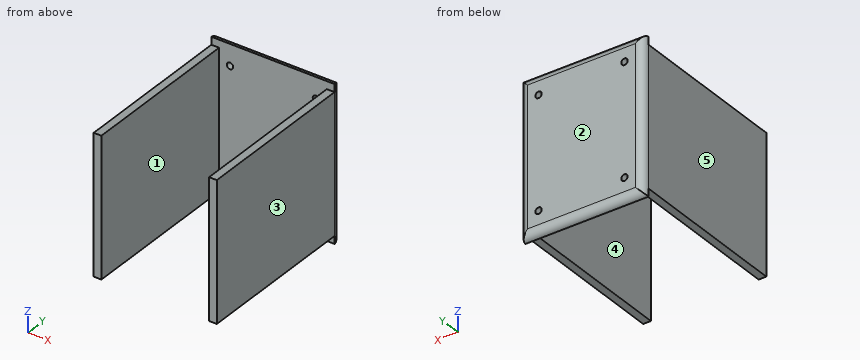
Autodesk Inventor part; units mm, degrees
ref_plane "YZ Plane" through (0, 0, 0) normal (1, 0, 0) x (0, 1, 0)
ref_plane "XZ Plane" through (0, 0, 0) normal (0, 1, 0) x (-1, 0, 0)
ref_plane "XY Plane" through (0, 0, 0) normal (0, 0, 1) x (1, 0, 0)
ref_plane "Plano de trabajo1" through (0, 3, 0) normal (0, 1, 0) x (1, 0, 0)
ref_plane "Plano de trabajo2" through (4.2498, 73, -5.25) normal (0, 1, 0) x (1, 0, 0)
sketch "Boceto3" plane through (4.2498, 73, -5.25) normal (0, 1, 0) x (1, 0, 0)
  line L0 (37.7502, 51.75) -> (40.7502, 51.75)
  line L1 (-7.2498, -8.25) -> (40.7502, -8.25)
  line L2 (40.7502, -8.25) -> (40.7502, 51.75)
  line L3 (40.7502, 51.75) -> (-7.2498, 51.75)
  line L4 (-7.2498, 51.75) -> (-7.2498, -8.25)
  circle A0 centre (33.5, 43.5) radius 1.25
  circle A1 centre (33.5, 0) radius 1.25
  circle A2 centre (0, 43.5) radius 1.25
  circle A3 centre (0, 0) radius 1.25
  point P0 (-4.2498, -5.25)
  point P1 (37.7502, -5.25)
  point P2 (37.7502, 48.75)
  dimension "d39" = 2.5
  dimension "d40" = 2.5
  dimension "d41" = 2.5
  dimension "d42" = 2.5
ref_plane "Plano de trabajo3" through (4.2498, 73, -5.25) normal (0, -1, 0) x (1, 0, 0)
sketch "Boceto5" plane through (4.2498, 73, -5.25) normal (0, -1, 0) x (1, 0, 0)
  line L0 (-4.2498, 5.25) -> (-4.2498, -48.75)
  line L1 (-4.2498, 5.25) -> (-4.2498, -48.75)
  line L2 (37.7502, -48.75) -> (37.7502, 5.25)
  line L3 (37.7502, 5.25) -> (37.7502, 8.25)
  line L4 (37.7502, -48.75) -> (37.7502, -51.75)
  line L5 (-4.2498, 5.25) -> (-7.2498, 5.25)
  line L6 (-4.2498, -48.75) -> (-7.2498, -48.75)
  line L7 (37.7502, -48.75) -> (40.7502, -48.75)
  line L8 (37.7502, 5.25) -> (40.7502, 5.25)
  line L9 (40.7502, 5.25) -> (40.7502, -48.75)
  line L10 (40.7502, -51.75) -> (40.7502, 8.25)
  line L11 (-7.2498, -48.75) -> (-7.2498, 5.25)
  line L12 (-7.2498, 8.25) -> (-7.2498, -51.75)
extrude "Extrusión5" add sketch "Boceto5" along normal blind 64
extrude "Extrusión6" add sketch "Boceto3" along normal blind 3
fillet "Empalme3" radius 3 4 edges at (21, 76, 3) (-3, 76, -27) (45, 76, -27) (21, 76, -57)
properties part number "Relé - columnes tapa"
Input: part model. Units: mm. Frame: model coordinates. Face numbers are marked on the shaded views. A direction names the side the tool comes from. Round coordinates to 2 decimals unless told otherwise and drop trailing zeros. Order: outer loops, then holes, each group sorted by start corner. A loop starts at its lowest first (then second) coordinate and runs counter-clockwise, first axis right, second up. Notation, with made-up numbers: (-12.5, 32) - (28.5, 32) arc R13 cw to (28.5, 39) - close; hole circle Ø5 at (49.5, 9.5). An arc over 180 degrees is marked (long way). Answer in a Markdown table with one row per item.
Item 1: Section query B-B (y = 20.5). Return the cut outline in (x, z), then the cut area to 3 significant figures.
Model answer:
| item | result |
|---|---|
| outline | (-3, -54) - (0, -54) - (0, 0) - (-3, 0) - close; (42, -54) - (45, -54) - (45, 0) - (42, 0) - close |
| area | 324 mm² |
Item 2: Section query A-A (z = -48.75). Return the cut outline in (x, y), then the cut area to 3 significant figures.
Model answer:
| item | result |
|---|---|
| outline | (-3, 9) - (0, 9) - (0, 73) - (3, 73) - (3, 76) - (0, 76) arc R3 ccw to (-3, 73) - close; (5.5, 73) - (36.5, 73) - (36.5, 76) - (5.5, 76) - close; (39, 73) - (42, 73) - (42, 9) - (45, 9) - (45, 73) arc R3 ccw to (42, 76) - (39, 76) - close |
| area | 509 mm² |
Item 3: Reachability of the marked faces 1 and 2 from +Z, -Z, +X, -X, +Y, -Y: full face, straight path, thin tool, end or side. Return the list, or none.
Model answer:
| item | result |
|---|---|
| face 1 | +Z, -Z, -Y |
| face 2 | +Z, -Z, +X, -X, +Y |
Item 4: Pin query (flat end, axial travel): pin 1 (6 mm diameter, centred on x = 2.5, y = 62, fed in from +Z); pin 2 (2.5 mm diameter, centred on x = 43, y = 57, fed in from -Z); pin 3 (2 mm diameter, centred on x = 4.25, z = -48.75, fed in from +Y); pin 4 (3 mm diameter, centred on x = 37.75, z = -5.25, fed in from -Y). Return the tip coordinate at first contact, or that it passes through.
Model answer:
| item | result |
|---|---|
| pin 1 | stops at z = 0 |
| pin 2 | stops at z = -54 |
| pin 3 | passes through |
| pin 4 | stops at y = 73 |
Item 5: Mould query, pull axis X, two halves, no side actions, for the marked faces 3, 4 and 5. Classes: released by +X, released by -X, zero draft, split by the parting line, or undercut.
Model answer:
| item | result |
|---|---|
| face 3 | released by +X |
| face 4 | undercut |
| face 5 | released by -X |
Item 6: Line query: line 1 (X direction, y = 20, z = -25); line 2 (X direction, y = 74.1, z = -5.25); line 3 (X direction, y = 75, z = -5.25). Output: solid intervals per line, ascending.
Model answer:
| item | result |
|---|---|
| line 1 | x = -3 to 0, 42 to 45 |
| line 2 | x = -2.79 to 3, 5.5 to 36.5, 39 to 44.79 |
| line 3 | x = -2.24 to 3, 5.5 to 36.5, 39 to 44.24 |
Item 7: Section query D-D (z = -15.5). Return the cut outline in (x, y), then the cut area to 3 significant figures.
Model answer:
| item | result |
|---|---|
| outline | (-3, 9) - (0, 9) - (0, 73) - (42, 73) - (42, 9) - (45, 9) - (45, 73) arc R3 ccw to (42, 76) - (0, 76) arc R3 ccw to (-3, 73) - close |
| area | 524 mm² |
